Autodesk Inventor part; units mm, degrees
ref_plane "YZ Plane" through (0, 0, 0) normal (1, 0, 0) x (0, 1, 0)
ref_plane "XZ Plane" through (0, 0, 0) normal (0, 1, 0) x (-1, 0, 0)
ref_plane "XY Plane" through (0, 0, 0) normal (0, 0, 1) x (1, 0, 0)
sketch "Sketch1" plane through (0, 0, 0) normal (0, 0, 1) x (1, 0, 0)
  arc A0 (-54.4767, 14.3972) -> (-15, 60) centre (-62.8769, 61.5571) ccw
  arc A1 (-49.5719, -5) -> (-54.4767, 14.3972) centre (-74.5236, -0.9906) ccw
  line L0 (-49.5719, -5) -> (-20, -5)
  arc A2 (-16, -9) -> (-20, -5) centre (-20, -9) ccw
  line L1 (-16, -9) -> (-16, -20.3999)
  line L2 (-16, -20.3999) -> (-13.5, -21.5)
  line L3 (-13.5, -21.5) -> (-16, -25.9706)
  line L4 (-16, -25.9706) -> (-16, -67)
  line L5 (-16, -67) -> (0, -67)
  line L6 (0, -67) -> (0, 65)
  line L7 (0, 65) -> (-15, 65)
  line L8 (-15, 65) -> (-15, 60)
  circle A3 centre (-8, 50) radius 5.25
  circle A4 centre (-8, -55.4085) radius 5.25
  arc A5 (-54.4767, 14.3972) -> (-15, 60) centre (-62.8769, 61.5571) ccw
  arc A6 (-49.5719, -5) -> (-54.4767, 14.3972) centre (-74.5236, -0.9906) ccw
  line L9 (-49.5719, -5) -> (-20, -5)
  arc A7 (-16, -9) -> (-20, -5) centre (-20, -9) ccw
  line L10 (-16, -9) -> (-16, -20.3999)
  line L11 (-16, -20.3999) -> (-13.5, -21.5)
  line L12 (-13.5, -21.5) -> (-16, -25.9706)
  line L13 (-16, -25.9706) -> (-16, -67)
  line L14 (-16, -67) -> (0, -67)
  line L15 (0, -67) -> (0, 65)
  line L16 (0, 65) -> (-15, 65)
  line L17 (-15, 65) -> (-15, 60)
  circle A8 centre (-8, 50) radius 5.25
  circle A9 centre (-8, -55.4085) radius 5.25
  point P0 (0, 0)
extrude "Extrusion1" add sketch "Sketch1" along normal blind 4.7625
properties part number "1-4inch_FixedKnifeBig_Piece1"
The model under review builds one solid part; all positions refer to its coordinate system, in mm. A direction names the side the tool comes from. Round coordinates to 2 decimals unless told otherwise and drop trailing zeros. Loops run counter-clockwise (first coordinate to the right, second up) from the corner with the lowest first, then second, coordinate; pieces in that order, holes last. Notation, with made-up numbers: (50, 15.5) -> (60, 15.5) arc R26 ccw to (60, 35.5) -> close; hole circle Ø3 at (84, 69). An arc over 180 degrees is marked (long way). Answer as a JSON object with one key per item and string values. Group by question number.
1) For pin 1 Ø1.4 at (x, z) = (-40, 2) entering from -Y; pin 2 Ø1.4 at (y, z) = (-12.5, 1.5) entering from -X; pin 3 Ø17 at (x, y) = (-8, -55.41) entering from -Z, all flat-tipped, find the tip position at first contact; note any pin that passes through.
2) For faces 4 (the face through (-15, 63, 2)), 5 (the face through (-14.77, -20.94, 2.35)), 6 (the face through (-8, -67, 2)), 7 (the face through (-16, -46, 2)), list the 3-axis set-ups (+Z, -Z, +X, -X, +Y, -Y) from which the entire face can be reached by the end or side of a thin tool; tool diameter is ignored.
3) For line 1 (Y direction, x = -8, z = 3.1); line 2 (Y direction, x = -4, z = 0.3); line 3 (X direction, y = -34.5, z = 0.6), list the stretches that pass through material, from the lowest coordinate up. Write a range as [from, to].
4) We need section C-C on z = 3.7. Write out the cut boundary in (x, y), then the cut area to 3 significant figures.
5) We need section D-D on y = -42.5. Write out the cut boundary in (x, z).
6) We need section B-B on y = 50. Write out the cut boundary in (x, z), then the cut area to 4 significant figures.
7) Mouldability with a two-part tool opening along X and no side actions: class faces 1 (the face through (-17.203, -6.141, 2.348)), 2 (the face through (-5.18, 45.57, 2.35)), 3 (the face through (-7, 65, 2)) as released by +X, released by -X, zero draft, split by the parting line, or undercut.
8) We need section A-A on x = -8. Write out the cut boundary in (y, z).
Result set:
{
 "1": {"pin 1": "y = -5", "pin 2": "x = -16", "pin 3": "z = 0"},
 "2": {"face 4": "+Z, -Z, -X, +Y", "face 5": "+Z, -Z, -X", "face 6": "+Z, -Z, +X, -X, -Y", "face 7": "+Z, -Z, -X, -Y"},
 "3": {"line 1": "[-67, -60.66], [-50.16, 44.75], [55.25, 65]", "line 2": "[-67, -58.81], [-52.01, 46.6], [53.4, 65]", "line 3": "[-16, 0]"},
 "4": {"outline": "(-54.48, 14.4) arc R25.27 cw to (-49.57, -5) -> (-20, -5) arc R4 cw to (-16, -9) -> (-16, -20.4) -> (-13.5, -21.5) -> (-16, -25.97) -> (-16, -67) -> (0, -67) -> (0, 65) -> (-15, 65) -> (-15, 60) arc R47.9 cw to start; hole circle Ø10.5 at (-8, -55.41); hole circle Ø10.5 at (-8, 50)", "area": "3,020 mm²"},
 "5": {"outline": "(-16, 0) -> (0, 0) -> (0, 4.76) -> (-16, 4.76) -> close"},
 "6": {"outline": "(-16.39, 0) -> (-13.25, 0) -> (-13.25, 4.76) -> (-16.39, 4.76) -> close; (-2.75, 0) -> (0, 0) -> (0, 4.76) -> (-2.75, 4.76) -> close", "area": "28.05 mm²"},
 "7": {"face 1": "released by -X", "face 2": "undercut", "face 3": "zero draft"},
 "8": {"outline": "(-67, 0) -> (-60.66, 0) -> (-60.66, 4.76) -> (-67, 4.76) -> close; (-50.16, 0) -> (44.75, 0) -> (44.75, 4.76) -> (-50.16, 4.76) -> close; (55.25, 0) -> (65, 0) -> (65, 4.76) -> (55.25, 4.76) -> close"}
}
